from build123d import *

# Parameters (mm, degrees)
SKETCH1_W           = 26
SKETCH1_H           = 42
BOSS_EXTRUDE1_DEPTH = 3
SKETCH4_R           = 3.4
SKETCH4_R_2         = 1.9
BOSS_EXTRUDE2_DEPTH = 9


with BuildPart() as part:
    # Sketch1 → Boss-Extrude1 (new body)
    with BuildSketch(Plane(origin=(0, 0, 0), x_dir=(1, 0, 0), z_dir=(0, 1, 0))):
        with Locations((-3.575345375, -3.834293295)):
            Rectangle(SKETCH1_W, SKETCH1_H)
    extrude(amount=BOSS_EXTRUDE1_DEPTH)

    # Sketch4 → Boss-Extrude2 (add)
    # profile 1 of 2: a face of its own
    with BuildSketch(Plane.XZ):
        with Locations(Location((-6.825345375, 7.834293295, 0), (0, 0, 90))):
            Circle(SKETCH4_R)
        with Locations(Location((-6.825345375, 7.834293295, 0), (0, 0, 270))):
            Circle(SKETCH4_R_2, mode=Mode.SUBTRACT)
    # profile 2 of 2: a face of its own
    with BuildSketch(Plane.XZ):
        with Locations(Location((2.924654625, -9.915706705, 0), (0, 0, 90))):
            Circle(SKETCH4_R)
        with Locations(Location((2.924654625, -9.915706705, 0), (0, 0, 270))):
            Circle(SKETCH4_R_2, mode=Mode.SUBTRACT)
    extrude(amount=BOSS_EXTRUDE2_DEPTH)


solid = part.part
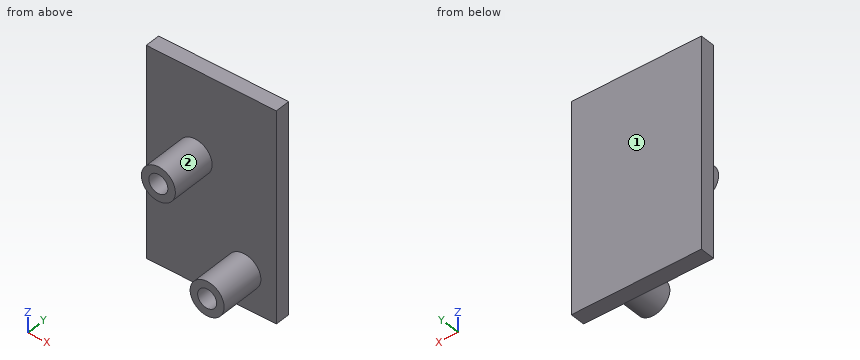
Check sheet for the modelled part. Datum: model origin and axes. Units: mm. Face numbers are marked on the shaded views. A direction names the side the tool comes from. Give positions to 0.01 mm unless a question says otherwise; leave off trailing zeros. Loops run counter-clockwise (first coordinate to the right, second up) from the corner with the lowest first, then second, coordinate; pieces in that order, holes last. Notation, with made-up numbers: M 59.5,76 L 94.5,76 A32 cw 94.5,104 Z; hole C 82.5,59 d10. An arc over 180 degrees is marked long. Answer as a JSON object with one key per item and string values. Group by question number.
Q1. Go/stop test with flat-tipped pins: P1, Ø3, axis at x = -6.5, z = 8.5, coming from the -Y side; P2, Ø1.5, axis at x = -6.5, y = -3.5, coming from the -Z side; P3, Ø6, axis at x = -4, z = 20, coming from the -Y side; P4, Ø3, axis at y = -6.5, z = -5.5, coming from the -X side. Record where each tip stops, or that it passes through.
Q2. Material ranges on line 1 along Y through (x, z) = (-0.5, -12); line 2 along Z through (x, y) = (2.5, -8); line 3 along X through (y, z) = (-5.5, -13), recorded low to high. Write a range as [from, to].
Q3. Access from +Z, -Z, +X, -X, +Y, -Y to the whole of each face (thin tool, end or side, straight path). Record for the marked faces 1 and 2.
Q4. Cross-section at A-A on x = -6.25. Record the cut outline in (y, z).
Q5. Cross-section at C-C on z = -12.5. Record the cut outline in (x, y), then the cut area to 3 significant figures.
Q6. Cross-section at B-B on y = -7.5. Record the cut outline in (x, z).
Q7. Cross-section at D-D on x = 5.25. Record the cut outline in (y, z), then the cut area to 3 significant figures.
Evaluation:
{
 "1": {"P1": "stops at y = -9", "P2": "stops at z = 4.43", "P3": "stops at y = 0", "P4": "stops at x = 1.18"},
 "2": {"line 1": "y = [0, 3]", "line 2": "z = [-13.29, -11.77], [-8.06, -6.54]", "line 3": "x = [1.49, 4.36]"},
 "3": {"face 1": "+Z, -Z, +X, -X, +Y", "face 2": "-Y"},
 "4": {"outline": "M -9,4.48 L 0,4.48 L 0,-17.17 L 3,-17.17 L 3,24.83 L 0,24.83 L 0,11.19 L -9,11.19 L -9,9.65 L 0,9.65 L 0,6.02 L -9,6.02 Z"},
 "5": {"outline": "M -16.58,0 L 0.72,0 L 0.72,-9 L 5.13,-9 L 5.13,0 L 9.42,0 L 9.42,3 L -16.58,3 Z", "area": "118 mm2"},
 "6": {"outline": "C -6.83,7.83 d6.8; C 2.92,-9.92 d6.8; hole C -6.83,7.83 d3.8; hole C 2.92,-9.92 d3.8"},
 "7": {"outline": "M -9,-12.4 L 0,-12.4 L 0,-17.17 L 3,-17.17 L 3,24.83 L 0,24.83 L 0,-7.44 L -9,-7.44 Z", "area": "171 mm2"}
}
